Work out the finished part from the listing and answer in its coordinate system (mm). Face numbers are marked on the shaded views. Round coordinates to 2 decimals unless told otherwise and drop trailing zeros. Loops run counter-clockwise (first coordinate to the right, second up) from the corner with the lowest first, then second, coordinate; pieces in that order, holes last. Notation, with made-up numbers: (8, 84) - (20, 84) arc R13 ccw to (20, 93) - close; hole circle Ø10 at (51.25, -25.75). An arc over 180 degrees is marked (long way). Answer as CSV lines item,"result". Start each with the question number.
```python
from build123d import *

# Parameters (mm, degrees)
F0_W     = 50
F0_H     = 50
F0_R     = 10.5
F1_DEPTH = 3
F4_R     = 2
F5_SIZE  = 1


with BuildPart() as f1:
    # F0 (on Top) → F1 (new body)
    with BuildSketch(Plane.XY):
        Rectangle(F0_W, F0_H)
        Circle(F0_R, mode=Mode.SUBTRACT)
    extrude(amount=F1_DEPTH)

    # F2 (on Front) → F3 (revolve)
    with BuildSketch(Plane.XZ):
        with BuildLine():
            Line((-10.5, 3), (-10.5, 53))
            Line((-10.5, 53), (-13.5, 53))
            Line((-13.5, 53), (-13.5, 50.842942))
            Line((-13.5, 50.842942), (-13, 50.842942))
            Line((-13, 50.842942), (-13.5, 45.818362))
            Line((-13.5, 45.818362), (-13.506682, 45.019927))
            Line((-13.506682, 45.019927), (-13.006682, 45.019927))
            Line((-13.006682, 45.019927), (-13.506682, 39.995346))
            Line((-13.506682, 39.995346), (-13.513363, 39.196911))
            Line((-13.513363, 39.196911), (-13.013363, 39.196911))
            Line((-13.013363, 39.196911), (-13.5, 34.306619))
            Line((-13.5, 34.306619), (-13.5, 33.373896))
            Line((-13.5, 33.373896), (-13.020045, 33.373896))
            Line((-13.020045, 33.373896), (-13.5, 28.550748))
            Line((-13.5, 28.550748), (-13.5, 27.550881))
            Line((-13.5, 27.550881), (-13.026726, 27.550881))
            Line((-13.026726, 27.550881), (-13.5, 22.794877))
            Line((-13.5, 22.794877), (-13.5, 8))
            ThreePointArc((-13.5, 8), (-14.964466, 4.464466), (-18.5, 3))
            Line((-18.5, 3), (-10.5, 3))
        make_face()
    revolve(axis=Axis((0, 0, 16.531735), (0, 0, -1)))

    # F4
    f4_edges = [f1.edges().sort_by_distance(p)[0] for p in [
        (13.5, 0, 53),
    ]]
    fillet(f4_edges, radius=F4_R)

    # F5
    f5_edges = [f1.edges().sort_by_distance(p)[0] for p in [
        (-25, 0, 3),
        (0, -25, 3),
        (25, 0, 3),
        (0, 25, 3),
        (-25, -25, 1.5),
        (25, -25, 1.5),
        (25, 25, 1.5),
        (-25, 25, 1.5),
    ]]
    chamfer(f5_edges, length=F5_SIZE)


solid = f1.part
```
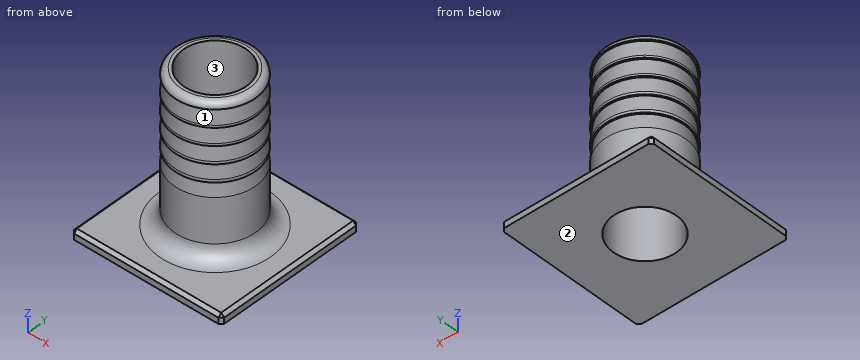
Item 1: Find the intervals of material crossed by L1, parallel to Y at x = 0, z = 15.5; L2, parallel to Z at x = 18.5, y = 5; L3, parallel to X at y = 0, z = 38, in increasing order.
Item 2: Section B-B, the plane z = 17.5 is taken. Give the vertices of the cut face in (x, y), and give its area (3 significant figures).
Item 3: Determine the mould class of the marked faces 1, 2 and 3 for opening direction X: pulls with the +X half, pulls with the -X half, needs draft (parallel to the pull), parting line crosses it, or undercut.
Item 4: Section A-A, the plane z = 49.5 is taken. Give the vertices of the cut face in (x, y), and give its area (3 significant figures).
Item 5: Flat-ended cylindrical pins translate along their axes: pin 1 Ø8 at (x, z) = (-7.5, 21.5) entering from +Y; pin 2 Ø12 at (x, z) = (-15, 44.5) entering from -Y; pin 3 Ø5 at (y, z) = (9, 11) entering from +X. Find the tip coordinate at first contact, or state that the pin passes through.
Answer:
1,L1,"y = -13.5 to -10.5, 10.5 to 13.5"
1,L2,"z = 0 to 3"
1,L3,"x = -13.13 to -10.5, 10.5 to 13.13"
2,outline,"circle Ø27 at (0, 0); hole circle Ø21 at (0, 0)"
2,area,"226 mm²"
3,face 1,"parting line crosses it"
3,face 2,"needs draft"
3,face 3,"undercut"
4,outline,"circle Ø26.27 at (0, 0); hole circle Ø21 at (0, 0)"
4,area,"196 mm²"
5,pin 1,"stops at y = 13.04"
5,pin 2,"stops at y = -10.05"
5,pin 3,"stops at x = 11.83"
